from build123d import *

# Parameters (mm, degrees)
EXTRUDE_1_DEPTH       = 60
SHEET_METAL_1_DEPTH   = 60
SHEET_METAL_1_2_DEPTH = 60
CUT_EXTRUDE_1_REACH   = 68.591
SKETCH_2_R            = 3.75
FILLET_1_R            = 2


# Read off the part's stored shape, not the designer's step: Преобразовать-Твердое тело1
with BuildPart() as part:
    # Sketch 1 → Бобышка-Вытянуть1 (new body)
    with BuildSketch(Plane.XY):
        Polygon((-12.5, 2), (12.5, 2), (12.5, 24.983479724), (14.5, 24.983479724), (14.5, 0), (-14.5, 0), (-14.5, 24.983479724), (-12.5, 24.983479724), align=None)
    extrude(amount=EXTRUDE_1_DEPTH)

    # Sheet Metal 1 outline → Sheet Metal 1 (cut)
    with BuildSketch(Plane.XY):
        with BuildLine():
            Line((-14.5, 0), (-10.5, 0))
            ThreePointArc((-10.5, 0), (-13.328427125, 1.171572875), (-14.5, 4))
            Line((-14.5, 4), (-14.5, 0))
        make_face()
        with BuildLine():
            ThreePointArc((14.5, 4), (13.328427125, 1.171572875), (10.5, 0))
            Line((10.5, 0), (14.5, 0))
            Line((14.5, 0), (14.5, 4))
        make_face()
    extrude(amount=SHEET_METAL_1_DEPTH, mode=Mode.SUBTRACT)

    # Sheet Metal 1 2 outline → Sheet Metal 1 2 (add)
    with BuildSketch(Plane.XY):
        with BuildLine():
            Line((-12.5, 2), (-10.5, 2))
            ThreePointArc((-10.5, 2), (-11.914213562, 2.585786438), (-12.5, 4))
            Line((-12.5, 4), (-12.5, 2))
        make_face()
        with BuildLine():
            ThreePointArc((12.5, 4), (11.914213562, 2.585786438), (10.5, 2))
            Line((10.5, 2), (12.5, 2))
            Line((12.5, 2), (12.5, 4))
        make_face()
    extrude(amount=SHEET_METAL_1_2_DEPTH)

    # Sketch 2 → Вырез-Вытянуть1 (cut, up to next)
    with BuildSketch(Plane.XZ, mode=Mode.PRIVATE) as cut_extrude_1_sk1:
        with Locations(Location((0, 45, 0), (0, 0, 270))):
            Circle(SKETCH_2_R)
    cut_extrude_1_tool1 = extrude(cut_extrude_1_sk1.sketch, amount=-CUT_EXTRUDE_1_REACH, mode=Mode.PRIVATE) & part.part
    # Sketch 2 → Вырез-Вытянуть1 (cut, up to next)
    with BuildSketch(Plane.XZ, mode=Mode.PRIVATE) as cut_extrude_1_sk2:
        with Locations(Location((0, 15, 0), (0, 0, 270))):
            Circle(SKETCH_2_R)
    cut_extrude_1_tool2 = extrude(cut_extrude_1_sk2.sketch, amount=-CUT_EXTRUDE_1_REACH, mode=Mode.PRIVATE) & part.part
    add(cut_extrude_1_tool1.solids().sort_by_distance((0, 0, 45))[0], mode=Mode.SUBTRACT)
    add(cut_extrude_1_tool2.solids().sort_by_distance((0, 0, 15))[0], mode=Mode.SUBTRACT)

    # Скругление1
    fillet_1_edges = [part.edges().sort_by_distance(p)[0] for p in [
        (13.5, 24.983479724, 60),
        (-13.5, 24.983479724, 60),
    ]]
    fillet(fillet_1_edges, radius=FILLET_1_R)


solid = part.part
Input: part model. Units: mm. Frame: model coordinates. A direction names the side the tool comes from. Coordinates: 2 decimals unless noted, no trailing zeros. Order: outer loops, then holes, each group sorted by start corner. A loop starts at its lowest first (then second) coordinate and runs counter-clockwise, first axis right, second up.
1. Cut plane C-C, the plane z = 15. Return loops of the section in (x, y).
Checked values:
outline: (-14.5, 4) arc R4 ccw to (-10.5, 0) - (-3.75, 0) - (-3.75, 2) - (-10.5, 2) arc R2 cw to (-12.5, 4) - (-12.5, 24.98) - (-14.5, 24.98) - close; (3.75, 0) - (10.5, 0) arc R4 ccw to (14.5, 4) - (14.5, 24.98) - (12.5, 24.98) - (12.5, 4) arc R2 cw to (10.5, 2) - (3.75, 2) - close
2. Ray query, line 1 along X through (y, z) = (21, 45.5); line 2 along Y through (x, z) = (10.25, 31); line 3 along X through (y, z) = (1.3, 45). Return the intervals inside material, ascending.
Checked values:
line 1: x = -14.5 to -12.5, 12.5 to 14.5
line 2: y = 0 to 2
line 3: x = -13.45 to -3.75, 3.75 to 13.45
3. Access query for faces 1 (the cylindrical face through (11.93, 2.6, 29.58)), 2 (the cylindrical face through (0.165, 0.986, 18.746)). Directions: +Z, -Z, +X, -X, +Y, -Y. A direction counts if a zero-diameter tool reaches every point of the face in a straight line with its end or side. Return the directions, or none.
Checked values:
face 1: +Z, -Z, +Y
face 2: +Y, -Y
4. Cut plane B-B, the plane x = 0. Return loops of the section in (y, z), plus the area to 3 significant figures.
Checked values:
outline: (0, 0) - (2, 0) - (2, 11.25) - (0, 11.25) - close; (0, 18.75) - (2, 18.75) - (2, 41.25) - (0, 41.25) - close; (0, 48.75) - (2, 48.75) - (2, 60) - (0, 60) - close
area: 90.0 mm2
5. Draft query along X for faces 3 (the cylindrical face through (13.51, 24.38, 59.43)), 4 (the flat face through (14.5, 15, 30)), 5 (the flat face through (12.5, 14, 30)). Return one class per face: +X half, -X half, draft (parallel to the pull), parting line (faces both ways), or undercut.
Checked values:
face 3: draft
face 4: +X half
face 5: undercut
6. Cut plane A-A, the plane y = 8.75. Return loops of the section in (x, z), plus the area to 3 significant figures.
Checked values:
outline: (-14.5, 0) - (-12.5, 0) - (-12.5, 60) - (-14.5, 60) - close; (12.5, 0) - (14.5, 0) - (14.5, 60) - (12.5, 60) - close
area: 240 mm2
7. Cut plane D-D, the plane z = 29. Return loops of the section in (x, y).
Checked values:
outline: (-14.5, 4) arc R4 ccw to (-10.5, 0) - (10.5, 0) arc R4 ccw to (14.5, 4) - (14.5, 24.98) - (12.5, 24.98) - (12.5, 4) arc R2 cw to (10.5, 2) - (-10.5, 2) arc R2 cw to (-12.5, 4) - (-12.5, 24.98) - (-14.5, 24.98) - close
